Autodesk Inventor part; units mm, degrees
ref_plane "Work Plane1" through (0, 0, 0) normal (1, 0, 0) x (0, 1, 0)
ref_plane "Work Plane2" through (0, 1, 16.53) normal (0, 1, 0) x (1, 0, 0)
ref_plane "XZ Plane" through (0, 0, 0) normal (0, 1, 0) x (-1, 0, 0)
sketch "Sketch1" plane through (0, 0, 0) normal (0, 1, 0) x (-1, 0, 0)
  circle A0 centre (0, 27.06) radius 0.5
  circle A1 centre (0, 24.06) radius 0.5
  circle A2 centre (0, 16.53) radius 4.375
  circle A3 centre (0, 3) radius 0.5
  circle A4 centre (0, 6) radius 0.5
  circle A5 centre (0, 9) radius 0.5
  circle A6 centre (0, 0) radius 0.5
  circle A7 centre (0, 30.06) radius 0.5
  circle A8 centre (0, 33.06) radius 0.5
  circle A9 centre (0, 16.53) radius 19.18
extrude "Extrusion1" add sketch "Sketch1" along normal blind 1
sketch "Sketch5" plane through (0, 1, 16.53) normal (0, 1, 0) x (1, 0, 0)
  line L0 (4.875, 0) -> (4.875, -17.5)
  line L1 (4.875, -17.5) -> (6.875, -17.5)
  line L2 (6.875, -17.5) -> (6.875, 0)
  line L3 (4.875, 0) -> (4.875, 17.5)
  line L4 (4.875, 17.5) -> (6.875, 17.5)
  line L5 (6.875, 17.5) -> (6.875, 0)
  point P0 (0, 16.53)
extrude "Extrusion4" add sketch "Sketch5" along normal blind 12
sketch "Sketch6" plane through (4.875, 1, -0.97) normal (-1, 0, 0) x (0, 0, 1)
  line L0 (36.68, 0) -> (-1.68, 0)
  line L1 (35, 2) -> (17.5, 2)
  line L2 (17.5, 2) -> (0, 2)
  line L3 (0, 12) -> (35, 12)
  line L4 (35, 2) -> (35, 12)
  line L5 (0, 2) -> (0, 12)
  circle A0 centre (8.75, 7) radius 1.5
  circle A1 centre (26.25, 7) radius 1.5
  point P0 (0.97, -1)
  dimension "d18" = 3
extrude "Extrusion5" cut sketch "Sketch6" against normal blind 12 contours A0 | A1
extrude "Extrusion6" add sketch "Sketch6" along normal blind 2.375
ref_plane "Work Plane1" through (0, 0, 0) normal (1, 0, 0) x (0, 1, 0)
mirror "Mirror1" about plane through (0, 0, 0) normal (1, 0, 0) of "Extrusion6", "Extrusion4", "Extrusion5"
ref_plane "Work Plane2" through (0, 1, 16.53) normal (0, 1, 0) x (1, 0, 0)
sketch "Sketch7" plane through (0, 1, 16.53) normal (0, 1, 0) x (1, 0, 0)
  circle A0 centre (0, 0) radius 4.375
  circle A1 centre (0, 16.53) radius 0.5
  circle A2 centre (0, 13.53) radius 0.5
  circle A3 centre (0, 10.53) radius 0.5
  circle A4 centre (0, 7.53) radius 0.5
  circle A5 centre (0, -10.53) radius 0.5
  circle A6 centre (0, -16.53) radius 0.5
  circle A7 centre (0, -13.53) radius 0.5
  circle A8 centre (0, -7.53) radius 0.5
  circle A9 centre (0, 0) radius 19.18
  circle A10 centre (0, 0) radius 4.375
  circle A11 centre (7.53, 0) radius 0.5
  circle A12 centre (10.53, 0) radius 0.5
  circle A13 centre (13.53, 0) radius 0.5
  circle A14 centre (16.53, 0) radius 0.5
  circle A15 centre (0, -13.53) radius 0.5
  circle A16 centre (-7.53, 0) radius 0.5
  circle A17 centre (-10.53, 0) radius 0.5
  circle A18 centre (-13.53, 0) radius 0.5
  circle A19 centre (-16.53, 0) radius 0.5
extrude "Extrusion7" cut sketch "Sketch7" along normal mid plane 10 contours A11 | A12 | A13 | A14 | A16 | A17 | A18 | A19
properties part number "horn_fin_normal"
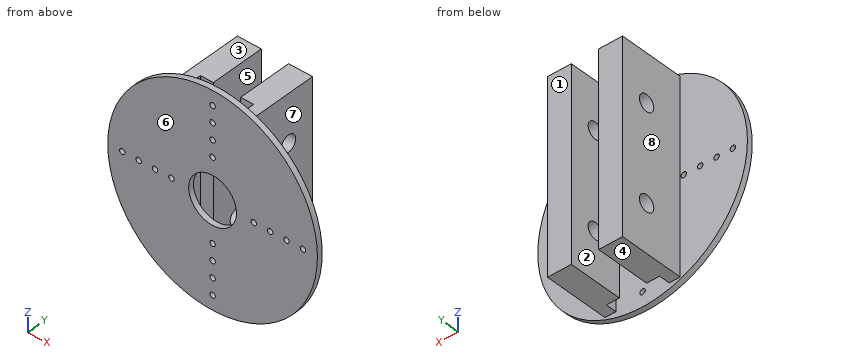
Check sheet for the modelled part. Datum: model origin and axes. Units: mm. Face numbers are marked on the shaded views. A direction names the side the tool comes from. Round coordinates to 2 decimals unless told otherwise and drop trailing zeros. Write each loop counter-clockwise with the first axis right and the second up, starting at its lowest first coordinate (ties: lowest second). Pieces come first, ordered by that corner, then holes. Notation, with made-up numbers: (74, 66.5) -> (102, 66.5) arc R23 cw to (102, 75.5) -> close; hole circle Ø9 at (-26, -40). An arc over 180 degrees is marked (long way). Answer as CSV lines item,"result". Start each with the question number.
1) Tool access check on the marked faces 1, 2, 3 and 4. Record the directions out of +Z, -Z, +X, -X, +Y, -Y that give a thin tool (end or side, any length) a straight path to the whole face; none if there is none.
2) Release check for a two-part mould opening along X. For the marked faces 5, 6, 7 and 8 record: pulls with the +X half, pulls with the -X half, needs draft (parallel to the pull), parting line crosses it, or undercut.
3) Go/stop test with flat-tipped pins: P1, Ø3.5, axis at y = 8, z = 25.28, coming from the +X side (3 decimals); P2, Ø3.5, axis at y = 6, z = 15.5, coming from the -X side (3 decimals); P3, Ø2.5, axis at y = 8, z = 7.78, coming from the +X side; P4, Ø1.3, axis at x = -4.5, y = 7.5, coming from the +Z side. Record where each tip stops, or that it passes through.
4) Section check A-A on y = 6. Enter the section's corners in (x, z) (3 decimals), and give its area (3 significant figures).
5) Section check C-C on z = 0. Enter the section's corners in (x, y) (3 decimals).
6) Section check D-D on y = 8. Enter the section's corners in (x, z) (3 decimals).
7) Material ranges on line 1 (Y direction, x = 3.7, z = 25.28); line 2 (X direction, y = 3.5, z = 19.5) (3 decimals); line 3 (Z direction, x = -3, y = 9), recorded low to high. Write a range as from..to.
8) Section check B-B on x = 13.53. Enter the section's corners in (y, z).
Found:
1,face 1,"+Z, -Z, +X, -X, +Y"
1,face 2,"+Z, -Z, +Y"
1,face 3,"+Z, +X, -X, +Y"
1,face 4,"-Z, +X, -X, +Y"
2,face 5,"undercut"
2,face 6,"needs draft"
2,face 7,"pulls with the +X half"
2,face 8,"pulls with the -X half"
3,P1,"stops at x = 6.875"
3,P2,"stops at x = -6.875"
3,P3,"passes through"
3,P4,"stops at z = 34.03"
4,outline,"(-6.875, -0.97) -> (-2.5, -0.97) -> (-2.5, 34.03) -> (-6.875, 34.03) -> close; (2.5, -0.97) -> (6.875, -0.97) -> (6.875, 34.03) -> (2.5, 34.03) -> close"
4,area,"306 mm^2"
5,outline,"(-9.728, 0) -> (-0.5, 0) -> (-0.5, 1) -> (-4.875, 1) -> (-4.875, 3) -> (-2.5, 3) -> (-2.5, 13) -> (-6.875, 13) -> (-6.875, 1) -> (-9.728, 1) -> close; (0.5, 0) -> (9.728, 0) -> (9.728, 1) -> (6.875, 1) -> (6.875, 13) -> (2.5, 13) -> (2.5, 3) -> (4.875, 3) -> (4.875, 1) -> (0.5, 1) -> close"
6,outline,"(-6.875, -0.97) -> (-2.5, -0.97) -> (-2.5, 6.28) -> (-6.875, 6.28) -> close; (-6.875, 9.28) -> (-2.5, 9.28) -> (-2.5, 23.78) -> (-6.875, 23.78) -> close; (-6.875, 26.78) -> (-2.5, 26.78) -> (-2.5, 34.03) -> (-6.875, 34.03) -> close; (2.5, -0.97) -> (6.875, -0.97) -> (6.875, 6.28) -> (2.5, 6.28) -> close; (2.5, 9.28) -> (6.875, 9.28) -> (6.875, 23.78) -> (2.5, 23.78) -> close; (2.5, 26.78) -> (6.875, 26.78) -> (6.875, 34.03) -> (2.5, 34.03) -> close"
7,line 1,"y = 0..1, 3..6.5, 9.5..13"
7,line 2,"x = -6.875..-2.5, 2.5..6.875"
7,line 3,"z = -0.97..6.66, 8.9..24.16, 26.4..34.03"
8,outline,"(0, 2.94) -> (1, 2.94) -> (1, 16.03) -> (0, 16.03) -> close; (0, 17.03) -> (1, 17.03) -> (1, 30.12) -> (0, 30.12) -> close"
